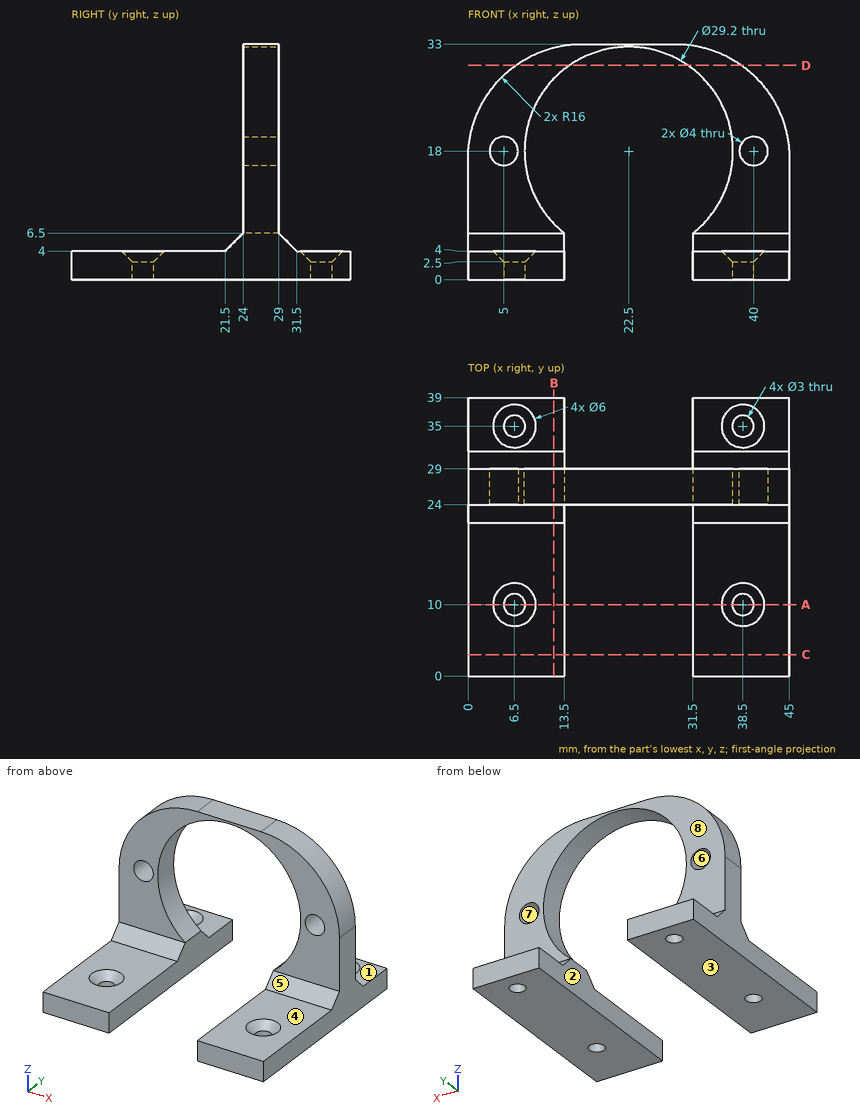
Source: three-view drawing plus pictorial views. Frame: mm from the lowest corner of the part. A direction names the side the tool comes from. Round coordinates to 2 decimals unless told otherwise and drop trailing zeros. Loops run counter-clockwise (first coordinate to the right, second up) from the corner with the lowest first, then second, coordinate; pieces in that order, holes last. Notation, with made-up numbers: M 41.5,19.5 L 54.5,19.5 A19 cw 54.5,37.5 Z; hole C 59.5,19.25 d11. An arc over 180 degrees is marked long. Answer as CSV lines item,"result". Start each with the question number.
(1) Reachability of the marked faces 1, 2, 3 and 4 from +Z, -Z, +X, -X, +Y, -Y: full face, straight path, thin tool, end or side. Return the list, or none.
(2) Section D-D, the plane z = 30. Output: boundary loops of the cut face in (x, y), plus the area to 3 significant figures.
(3) Section B-B, the plane x = 12. Output: boundary loops of the cut face in (y, z), plus the area to 3 significant figures.
(4) First-contact query: pin 1 (4 mm diameter, centred on x = 8.5, y = 17.5, fed in from +Z); pin 2 (8 mm diameter, centred on x = 4, y = 33.5, fed in from +Z); pin 3 (1 mm diameter, centred on x = 7, z = 11, fed in from +Y). Flat tips, straight axial feed; report the tip coordinate or a pass-through.
(5) Section C-C, the plane y = 3. Output: boundary loops of the cut face in (x, z), plus the area to 3 significant figures.
(6) Draft query along Z for the marked faces 5, 6, 7 and 8. Return one class per face: released by +Z, released by -Z, zero draft, split by the parting line, or undercut.
(7) Section A-A, the plane y = 10. Output: boundary loops of the cut face in (x, z), plus the area to 3 significant figures.
(8) Line query: line 1 (X direction, y = 10, z = 1); line 2 (Y direction, x = 6.5, z = 1.6); line 3 (Y direction, x = 40, z = 13). Output: solid intervals per line, ascending. Write a range as [from, to].
Values found:
1,face 1,"+Z, +X, -X, +Y"
1,face 2,"-Z, +Y, -Y"
1,face 3,"-Z, +X, -X, +Y, -Y"
1,face 4,"+Z, +X, -X, -Y"
2,outline,"M 6.67,24 L 14.18,24 L 14.18,29 L 6.67,29 Z; M 30.82,24 L 38.33,24 L 38.33,29 L 30.82,29 Z"
2,area,"75.1 mm²"
3,outline,"M 0,0 L 39,0 L 39,4 L 31.5,4 L 29,6.5 L 29,7.86 L 24,7.86 L 24,6.5 L 21.5,4 L 0,4 Z; M 24,28.14 L 29,28.14 L 29,32.49 L 24,32.49 Z"
3,area,"203 mm²"
4,pin 1,"stops at z = 4"
4,pin 2,"stops at z = 6"
4,pin 3,"stops at y = 29"
5,outline,"M 0,0 L 13.5,0 L 13.5,4 L 0,4 Z; M 31.5,0 L 45,0 L 45,4 L 31.5,4 Z"
5,area,"108 mm²"
6,face 5,"released by +Z"
6,face 6,"undercut"
6,face 7,"undercut"
6,face 8,"zero draft"
7,outline,"M 0,0 L 5,0 L 5,2.5 L 3.5,4 L 0,4 Z; M 8,0 L 13.5,0 L 13.5,4 L 9.5,4 L 8,2.5 Z; M 31.5,0 L 37,0 L 37,2.5 L 35.5,4 L 31.5,4 Z; M 40,0 L 45,0 L 45,4 L 41.5,4 L 40,2.5 Z"
7,area,"79.5 mm²"
8,line 1,"x = [0, 5], [8, 13.5], [31.5, 37], [40, 45]"
8,line 2,"y = [0, 8.5], [11.5, 33.5], [36.5, 39]"
8,line 3,"y = [24, 29]"
